```python
from build123d import *

# Parameters (mm, degrees)
F0_R     = 3.25
F0_R_2   = 14
F0_R_3   = 4
F0_R_4   = 1.7
F1_DEPTH = 7
F2_DEPTH = 5
F3_R     = 3.25
F3_R_2   = 1.7
F4_DEPTH = 4
F3_R_3   = 12.5077468671
F3_R_4   = 4
F5_DEPTH = 3
F6_SIZE  = 0.5


with BuildPart() as f1:
    # F0 (on Top) → F1 (new body)
    with BuildSketch(Plane.XY):
        with BuildLine():
            ThreePointArc((17.5, 12.4899959968), (14.8835536543, 15.5154706864), (11.7519612405, 18.0039275438))
            Line((11.7519612405, 18.0039275438), (-11.7519612405, 18.0039275438))
            ThreePointArc((-11.7519612405, 18.0039275438), (-14.8835536543, 15.5154706864), (-17.5, 12.4899959968))
            Line((-17.5, 12.4899959968), (-17.5, -12.4899959968))
            ThreePointArc((-17.5, -12.4899959968), (-14.8835536543, -15.5154706864), (-11.7519612405, -18.0039275438))
            Line((-11.7519612405, -18.0039275438), (11.7519612405, -18.0039275438))
            ThreePointArc((11.7519612405, -18.0039275438), (14.8835536543, -15.5154706864), (17.5, -12.4899959968))
            Line((17.5, -12.4899959968), (17.5, 12.4899959968))
        make_face()
        with Locations((-12.1975036036, -12.5487412054)):
            Circle(F0_R, mode=Mode.SUBTRACT)
        with Locations((12.5487412054, -12.1975036036)):
            Circle(F0_R, mode=Mode.SUBTRACT)
        with Locations((-12.5487412054, 12.1975036036)):
            Circle(F0_R, mode=Mode.SUBTRACT)
        Circle(F0_R_2, mode=Mode.SUBTRACT)
        with Locations((12.1975036036, 12.5487412054)):
            Circle(F0_R, mode=Mode.SUBTRACT)
        Circle(F0_R_2)
        Circle(F0_R_3, mode=Mode.SUBTRACT)
        with Locations((12.1975036036, 12.5487412054)):
            Circle(F0_R)
        with Locations((12.1975036036, 12.5487412054)):
            Circle(F0_R_4, mode=Mode.SUBTRACT)
        with Locations((-12.5487412054, 12.1975036036)):
            Circle(F0_R)
        with Locations((-12.5487412054, 12.1975036036)):
            Circle(F0_R_4, mode=Mode.SUBTRACT)
        with Locations((-12.1975036036, -12.5487412054)):
            Circle(F0_R)
        with Locations((-12.1975036036, -12.5487412054)):
            Circle(F0_R_4, mode=Mode.SUBTRACT)
        with Locations((12.5487412054, -12.1975036036)):
            Circle(F0_R)
        with Locations((12.5487412054, -12.1975036036)):
            Circle(F0_R_4, mode=Mode.SUBTRACT)
    extrude(amount=-F1_DEPTH)

    # F0 (on Top) → F2 (join)
    with BuildSketch(Plane.XY):
        Circle(F0_R_2)
        Circle(F0_R_3, mode=Mode.SUBTRACT)
    extrude(amount=F2_DEPTH)

    # F3 (on face) → F4 (cut)
    with BuildSketch(Plane(origin=(0, 0, -7), x_dir=(1, 0, 0), z_dir=(0, 0, -1))):
        with Locations((-12.1975036036, 12.5487412054)):
            Circle(F3_R)
        with Locations((-12.1975036036, 12.5487412054)):
            Circle(F3_R_2, mode=Mode.SUBTRACT)
        with Locations((12.5487412054, 12.1975036036)):
            Circle(F3_R)
        with Locations((12.5487412054, 12.1975036036)):
            Circle(F3_R_2, mode=Mode.SUBTRACT)
        with Locations((12.1975036036, -12.5487412054)):
            Circle(F3_R)
        with Locations((12.1975036036, -12.5487412054)):
            Circle(F3_R_2, mode=Mode.SUBTRACT)
        with Locations((-12.5487412054, -12.1975036036)):
            Circle(F3_R)
        with Locations((-12.5487412054, -12.1975036036)):
            Circle(F3_R_2, mode=Mode.SUBTRACT)
    extrude(amount=-F4_DEPTH, mode=Mode.SUBTRACT)

    # F3 (on face) → F5 (cut)
    with BuildSketch(Plane(origin=(0, 0, -7), x_dir=(1, 0, 0), z_dir=(0, 0, -1))):
        Circle(F3_R_3)
        Circle(F3_R_4, mode=Mode.SUBTRACT)
    extrude(amount=-F5_DEPTH, mode=Mode.SUBTRACT)

    # F6
    f6_edges = [f1.edges().sort_by_distance(p)[0] for p in [
        (-17.5, 0, 0),
        (-14.883554, -15.515471, 0),
        (0, -18.003928, -7),
        (14.883554, -15.515471, -7),
        (17.5, 0, -7),
        (14.883554, 15.515471, -7),
        (0, 18.003928, -7),
        (-14.883554, 15.515471, 0),
        (-12.507747, 0, -7),
        (-14, 0, 5),
        (14.883554, 15.515471, 0),
        (17.5, 0, 0),
        (14.883554, -15.515471, 0),
        (0, -18.003928, 0),
        (0, 18.003928, 0),
    ]]
    chamfer(f6_edges, length=F6_SIZE)


solid = f1.part
```
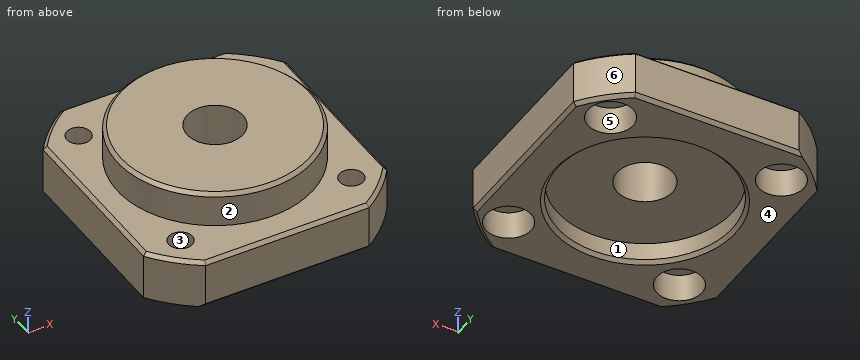
The listing builds one solid part. Answer for the finished solid, in the listing's coordinates (mm). Face numbers are marked on the shaded views. A direction names the side the tool comes from. Give positions to 0.01 mm unless a question says otherwise; leave off trailing zeros. Order: outer loops, then holes, each group sorted by start corner. A loop starts at its lowest first (then second) coordinate and runs counter-clockwise, first axis right, second up. Notation, with made-up numbers: (8.25, 73) - (45.25, 73) arc R35 ccw to (45.25, 109) - close; hole circle Ø4 at (89, 29). An arc over 180 degrees is marked (long way). Answer in a Markdown table with one row per item. Add a question column.
Q1. Find the intervals of material crossed by line 1 along X through (y, z) = (12, -3.25); line 2 along Y through (x, z) = (0, -4.45); line 3 along Z through (x, y) = (5, 5.5), in increasing order. Write a range as [from, to].
Q2. For a pull along Y with two mould halves and no side action, classify the marked faces 4, 5 and 6 as released by +Y, released by -Y, zero draft, split by the parting line, or undercut.
Q3. The part is cut by section A-A (x = 0). Determine the outline of the cut face in (y, z), then the cut area to 3 significant figures.
Q4. The part is cut by section B-B (y = 0). Determine the outline of the cut face in (x, z), then the cut area to 3 significant figures.
Q5. Given P1, Ø20, axis at x = 0, y = 0, coming from the -Z side; P2, Ø10, axis at x = 13, y = -9, coming from the -Z side; P3, Ø2.5, axis at x = -12.55, y = 12.2, coming from the -Z side; P4, Ø1, axis at x = 9, y = 12.5, coming from the +Z side, each flat-ended and moving along its own axis, determine where each tip first touches the part or whether it passes through.
Q6. Which of the six approach directions +Z, -Z, +X, -X, +Y, -Y give full straight-line access (tool end or side, diameter ignored) to the marked faces 1, 2 and 3?
Q7. The part is cut by section D-D (z = 3.75). Determine the outline of the cut face in (x, y), then the cut area to 3 significant figures.
Q8. The part is cut by section C-C (z = -1.5). Determine the outline of the cut face in (x, y), then the cut area to 3 significant figures.
Determined:
| question | item | result |
|---|---|---|
| 1 | line 1 | x = [-17.5, -15.79], [-9.3, 8.99], [15.4, 17.5] |
| 1 | line 2 | y = [-18, -12.51], [12.51, 18] |
| 1 | line 3 | z = [-4, 5] |
| 2 | face 4 | zero draft |
| 2 | face 5 | undercut |
| 2 | face 6 | released by +Y |
| 3 | outline | (-18, -6.5) - (-17.5, -7) - (-13.01, -7) - (-12.51, -6.5) - (-12.51, -4) - (-4, -4) - (-4, 5) - (-13.5, 5) - (-14, 4.5) - (-14, 0) - (-17.5, 0) - (-18, -0.5) - close; (4, -4) - (12.51, -4) - (12.51, -6.5) - (13.01, -7) - (17.5, -7) - (18, -6.5) - (18, -0.5) - (17.5, 0) - (14, 0) - (14, 4.5) - (13.5, 5) - (4, 5) - close |
| 3 | area | 244 mm² |
| 4 | outline | (-17.5, -7) - (-13.01, -7) - (-12.51, -6.5) - (-12.51, -4) - (-4, -4) - (-4, 5) - (-13.5, 5) - (-14, 4.5) - (-14, 0) - (-17, 0) - (-17.5, -0.5) - close; (4, -4) - (12.51, -4) - (12.51, -6.5) - (13.01, -7) - (17, -7) - (17.5, -6.5) - (17.5, -0.5) - (17, 0) - (14, 0) - (14, 4.5) - (13.5, 5) - (4, 5) - close |
| 4 | area | 237 mm² |
| 5 | P1 | stops at z = -4 |
| 5 | P2 | stops at z = -7 |
| 5 | P3 | passes through |
| 5 | P4 | stops at z = 0 |
| 6 | face 1 | -Z |
| 6 | face 2 | +Z |
| 6 | face 3 | +Z, -Z |
| 7 | outline | circle Ø28 at (0, 0); hole circle Ø8 at (0, 0) |
| 7 | area | 565 mm² |
| 8 | outline | (-17.5, -12.49) arc R21.5 ccw to (-11.75, -18) - (11.75, -18) arc R21.5 ccw to (17.5, -12.49) - (17.5, 12.49) arc R21.5 ccw to (11.75, 18) - (-11.75, 18) arc R21.5 ccw to (-17.5, 12.49) - close; hole circle Ø3.4 at (-12.55, 12.2); hole circle Ø3.4 at (-12.2, -12.55); hole circle Ø8 at (0, 0); hole circle Ø3.4 at (12.2, 12.55); hole circle Ø3.4 at (12.55, -12.2) |
| 8 | area | 1,120 mm² |
